from build123d import *

# Parameters (mm, degrees)
BOSS_EXTRUDE1_DEPTH            = 6.35
FILLET1_R                      = 1
SKETCH2_W                      = 7.5
SKETCH2_H                      = 3.15
CUT_EXTRUDE1_DEPTH             = 7.35
F_3_2_3_2_DIAMETER_HOLE1_D     = 3.2
F_3_2_3_2_DIAMETER_HOLE1_DEPTH = 6.35
F_3_2_3_2_DIAMETER_HOLE2_D     = 3.2
F_3_2_3_2_DIAMETER_HOLE2_DEPTH = 6.35


with BuildPart() as part:
    # Sketch1 → Boss-Extrude1 (new body)
    with BuildSketch(Plane(origin=(6.35, 0, 0), x_dir=(0, 0, -1), z_dir=(1, 0, 0))):
        Polygon((37.1, -7.95), (34.85, -7.95), (34.85, -1.4), (37.1, -1.4), (37.1, 0), (0, 0), (0, -1.4), (2.25, -1.4), (2.25, -7.95), (0, -7.95), (0, -9.35), (37.1, -9.35), align=None)
    extrude(amount=-BOSS_EXTRUDE1_DEPTH)

    # Fillet1
    fillet1_edges = [part.edges().sort_by_distance(p)[0] for p in [
        (3.175, -9.35, -37.1),
        (3.175, -9.35, 0),
        (3.175, 0, 0),
        (3.175, 0, -37.1),
    ]]
    fillet(fillet1_edges, radius=FILLET1_R)

    # Sketch2 → Cut-Extrude1 (cut, through all)
    with BuildSketch(Plane.ZY):
        with Locations((-18.55, -4.675)):
            Rectangle(SKETCH2_W, SKETCH2_H)
    extrude(amount=-CUT_EXTRUDE1_DEPTH, mode=Mode.SUBTRACT)

    # Ø3.2 (3.2) Diameter Hole1
    with Locations(Plane(origin=(6.35, 0, 0), x_dir=(0, 0, -1), z_dir=(1, 0, 0))):
        with Locations((28.55, -4.675)):
            Hole(F_3_2_3_2_DIAMETER_HOLE1_D / 2, depth=F_3_2_3_2_DIAMETER_HOLE1_DEPTH)

    # Ø3.2 (3.2) Diameter Hole2
    with Locations(Plane(origin=(6.35, 0, 0), x_dir=(0, 0, -1), z_dir=(1, 0, 0))):
        with Locations((8.55, -4.675)):
            Hole(F_3_2_3_2_DIAMETER_HOLE2_D / 2, depth=F_3_2_3_2_DIAMETER_HOLE2_DEPTH)


solid = part.part
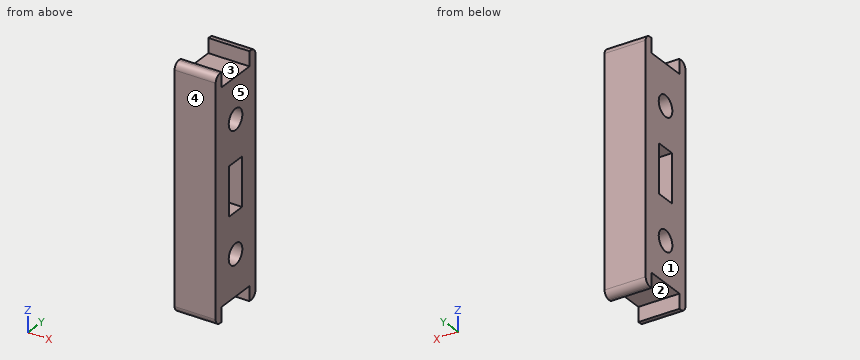
The listing builds one solid part. Answer for the finished solid, in the listing's coordinates (mm). Face numbers are marked on the shaded views. A direction names the side the tool comes from. Coordinates: 2 decimals unless noted, no trailing zeros. Loops run counter-clockwise (first coordinate to the right, second up) from the corner with the lowest first, then second, coordinate; pieces in that order, holes last. Notation, with made-up numbers: M -15.75,37.25 L 32.25,37.25 A23 ccw 32.25,73.25 Z; hole C -30,76 d1. An arc over 180 degrees is marked long. Answer in a Markdown table with one row per item.
1) Find section C-C (x = 1.75). Determine the outline of the cut face in (y, z) (3 decimals).
Answers below:
| item | result |
|---|---|
| outline | M -9.35,-36.1 A1 ccw -8.35,-37.1 L -7.95,-37.1 L -7.95,-34.85 L -1.4,-34.85 L -1.4,-37.1 L -1,-37.1 A1 ccw 0,-36.1 L 0,-1 A1 ccw -1,0 L -1.4,0 L -1.4,-2.25 L -7.95,-2.25 L -7.95,0 L -8.35,0 A1 ccw -9.35,-1 Z; hole C -4.675,-28.55 d3.2; hole C -4.675,-8.55 d3.2; hole M -6.25,-22.3 L -3.1,-22.3 L -3.1,-14.8 L -6.25,-14.8 Z |
2) Which of the six approach directions +Z, -Z, +X, -X, +Y, -Y give full straight-line access (tool end or side, diameter ignored) to the marked faces 1 and 2?
Answers below:
| item | result |
|---|---|
| face 1 | +Z, -Z, -X, +Y, -Y |
| face 2 | -Z, +X, -X |
3) Find section A-A (z = -16). Determine the outline of the cut face in (x, y), then the cut area to 3 significant figures.
Answers below:
| item | result |
|---|---|
| outline | M 0,-9.35 L 6.35,-9.35 L 6.35,-6.25 L 0,-6.25 Z; M 0,-3.1 L 6.35,-3.1 L 6.35,0 L 0,0 Z |
| area | 39.4 mm^2 |
4) Given pin 1 (2 mm diameter, centred on x = 5.5, y = -6, fed in from +Z); pin 2 (3 mm diameter, centred on y = -5, z = -15.5, fed in from -X); pin 3 (2.5 mm diameter, centred on x = 3.5, y = -4.5, fed in from -Z), each flat-ended and moving along its own axis, determine where each tip first touches the part or whether it passes through.
Answers below:
| item | result |
|---|---|
| pin 1 | z = -2.25 |
| pin 2 | x = 0 |
| pin 3 | z = -34.85 |
5) Find section D-D (z = -28.55). Determine the outline of the cut face in (x, y) (3 decimals), then the cut area to 3 significant figures.
Answers below:
| item | result |
|---|---|
| outline | M 0,-9.35 L 6.35,-9.35 L 6.35,-6.275 L 0,-6.275 Z; M 0,-3.075 L 6.35,-3.075 L 6.35,0 L 0,0 Z |
| area | 39.1 mm^2 |
6) Determine the mould class of the marked faces 3, 4 and 5 for opening direction Y: released by +Y, released by -Y, zero draft, split by the parting line, or undercut.
Answers below:
| item | result |
|---|---|
| face 3 | undercut |
| face 4 | released by -Y |
| face 5 | zero draft |
7) Find section B-B (y = -5.5). Determine the outline of the cut face in (x, z), then the cut area to 3 significant figures.
Answers below:
| item | result |
|---|---|
| outline | M 0,-34.85 L 6.35,-34.85 L 6.35,-29.92 L 0,-29.92 Z; M 0,-27.18 L 6.35,-27.18 L 6.35,-22.3 L 0,-22.3 Z; M 0,-14.8 L 6.35,-14.8 L 6.35,-9.92 L 0,-9.92 Z; M 0,-7.18 L 6.35,-7.18 L 6.35,-2.25 L 0,-2.25 Z |
| area | 125 mm^2 |
8) Find the intervals of material crossed by probe 1 along Y at (x, z) = (3.25, -8.55) (3 decimals); probe 2 along Y at (x, z) = (2.5, -2); probe 3 along Z at (x, y) = (1, -3.5), in increasing order.
Answers below:
| item | result |
|---|---|
| probe 1 | -9.35 to -6.275, -3.075 to 0 |
| probe 2 | -9.35 to -7.95, -1.4 to 0 |
| probe 3 | -34.85 to -29.64, -27.46 to -22.3, -14.8 to -9.64, -7.46 to -2.25 |
